Autodesk Inventor part; units mm, degrees
ref_plane "YZ Plane" through (0, 0, 0) normal (1, 0, 0) x (0, 1, 0)
ref_plane "XZ Plane" through (0, 0, 0) normal (0, 1, 0) x (-1, 0, 0)
ref_plane "XY Plane" through (0, 0, 0) normal (0, 0, 1) x (1, 0, 0)
sketch "Sketch1" plane through (0, 0, 0) normal (0, 1, 0) x (-1, 0, 0)
  circle A0 centre (0, 0) radius 4
  circle A1 centre (0, 0) radius 2.5
  circle A2 centre (0, 0) radius 2
  circle A3 centre (0, 0) radius 3.5
  dimension "d0" = 8
  dimension "d1" = 5
  dimension "d2" = 4
  dimension "d3" = 7
extrude "Extrusion1" add sketch "Sketch1" along normal blind 3 contours A0 | A1 | A3
extrude "Extrusion2" cut sketch "Sketch1" against normal blind 0.1 from surface at 3 contours A3
extrude "Extrusion3" cut sketch "Sketch1" along normal blind 0.1 contours A3
properties part number "Miniatur Kugellager MR 84 2RS 4x8x3 mm"
The model under review builds one solid part; all positions refer to its coordinate system, in mm. A direction names the side the tool comes from. Round coordinates to 2 decimals unless told otherwise and drop trailing zeros. Loops run counter-clockwise (first coordinate to the right, second up) from the corner with the lowest first, then second, coordinate; pieces in that order, holes last. Notation, with made-up numbers: (0, 18) -> (58, 18) arc R5 ccw to (58, 23) -> close; hole circle Ø1 at (16, 60). An arc over 180 degrees is marked (long way). One line per question, with ' | ' between items. Start each with the question number.
Item 1: Add section A-A, the plane x = 0. Write out the cut boundary in (y, z).
Item 2: Wall thickness on line 1 along Z through (x, y) = (0, 1.25); line 2 along Y through (x, z) = (-0.25, -3.25); line 3 along X through (y, z) = (0.65, -1): over which ranges is each line inside the solid? List them lowest first. Write a range as [from, to].
Item 3: Add section D-D, the plane z = -2.75. Write out the cut boundary in (x, y).
Item 4: For pin 1 (1.5 mm diameter, centred on x = 1, y = 2, fed in from +Z); pin 2 (1.5 mm diameter, centred on x = -2, y = 1.5, fed in from +Z); pin 3 (2.5 mm diameter, centred on x = 0, z = 0, fed in from -Y), all flat-tipped, find the tip position at first contact; note any pin that passes through.
Item 5: Add section C-C, the plane y = 1.7. Write out the cut boundary in (x, z), then the cut area to 3 significant figures.
Item 6: Add section B-B, the plane z = 0. Write out the cut boundary in (x, y).
Item 7: Draft analysis for pull direction X (two halves, no side actions). For faces 3 (the face through (1, 0, 2)), 4 (the face through (-2, 0.1, -2)), 5 (the face through (0.867, 1.479, 3.905)), state which applies: +X half, -X half, draft (parallel to the pull), parting line (faces both ways), or undercut.
Item 8: Machinability: for faces 1 (the face through (0, 1, 2)), 2 (the face through (-2, 2.9, -2)), which of the approach directions +Z, -Z, +X, -X, +Y, -Y give a long, thin tool a straight path to every point of the face, cutting with its end or side? Answer none if there is none.
Return value:
1) outline: (0, -4) -> (3, -4) -> (3, -3.5) -> (2.9, -3.5) -> (2.9, -2.5) -> (3, -2.5) -> (3, -2) -> (0, -2) -> (0, -2.5) -> (0.1, -2.5) -> (0.1, -3.5) -> (0, -3.5) -> close; (0, 2) -> (3, 2) -> (3, 2.5) -> (2.9, 2.5) -> (2.9, 3.5) -> (3, 3.5) -> (3, 4) -> (0, 4) -> (0, 3.5) -> (0.1, 3.5) -> (0.1, 2.5) -> (0, 2.5) -> close
2) line 1: z = [-4, -2], [2, 4] | line 2: y = [0.1, 2.9] | line 3: x = [-3.87, -1.73], [1.73, 3.87]
3) outline: (-2.9, 0) -> (-2.17, 0) -> (-2.17, 0.1) -> (2.17, 0.1) -> (2.17, 0) -> (2.9, 0) -> (2.9, 3) -> (2.17, 3) -> (2.17, 2.9) -> (-2.17, 2.9) -> (-2.17, 3) -> (-2.9, 3) -> close
4) pin 1: stops at z = 3.99 | pin 2: stops at z = 3.8 | pin 3: passes through
5) outline: circle Ø8 at (0, 0); hole circle Ø4 at (0, 0) | area: 37.7 mm2
6) outline: (-4, 0) -> (-3.5, 0) -> (-3.5, 0.1) -> (-2.5, 0.1) -> (-2.5, 0) -> (-2, 0) -> (-2, 3) -> (-2.5, 3) -> (-2.5, 2.9) -> (-3.5, 2.9) -> (-3.5, 3) -> (-4, 3) -> close; (2, 0) -> (2.5, 0) -> (2.5, 0.1) -> (3.5, 0.1) -> (3.5, 0) -> (4, 0) -> (4, 3) -> (3.5, 3) -> (3.5, 2.9) -> (2.5, 2.9) -> (2.5, 3) -> (2, 3) -> close
7) face 3: draft | face 4: undercut | face 5: parting line
8) face 1: +Y, -Y | face 2: +Y
